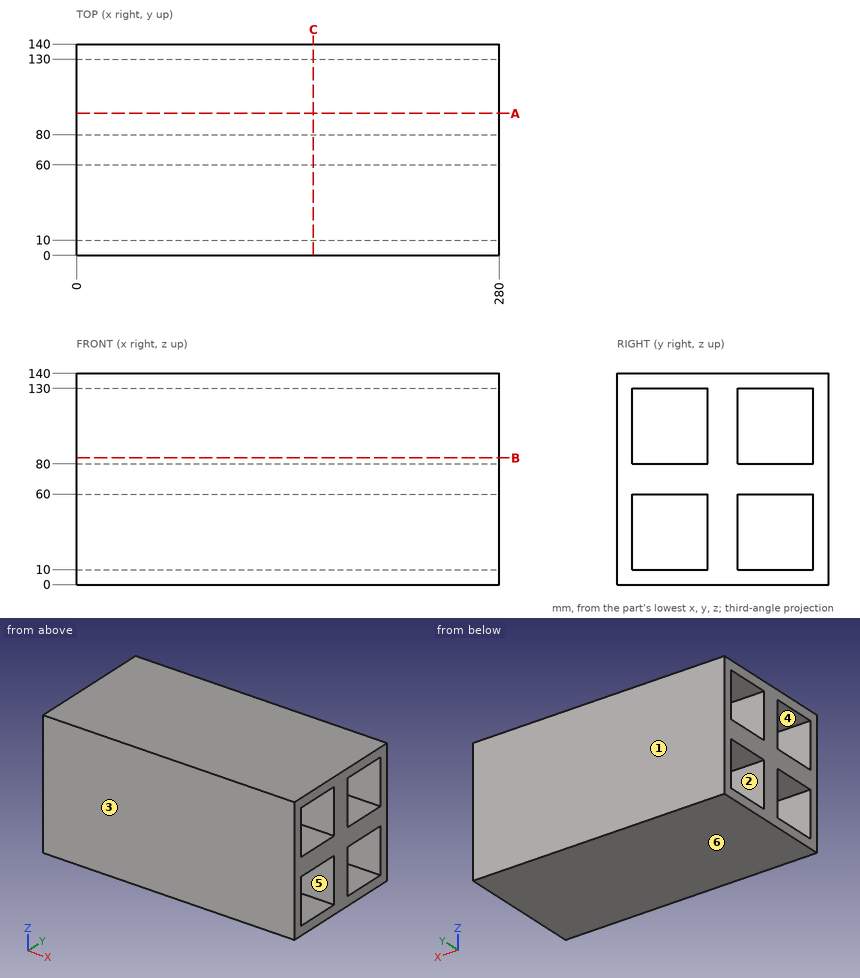
Study the drawing (mm; zero at the part's minimum x, y, z) and answer. A direction names the side the tool comes from. Give positions to 0.01 mm unless a question says otherwise; leave off trailing zeros. Write each loop counter-clockwise with the first axis right and the second up, starting at its lowest first coordinate (ties: lowest second). Pieces come first, ordered by that corner, then holes.
Item 1: Section C-C, the plane x = 157 is taken. Write down the section's boundary in (y, z), plus the area to 3 significant figures.
Item 2: Which of the six approach directions +Z, -Z, +X, -X, +Y, -Y give full straight-line access (tool end or side, diameter ignored) to the marked faces 1 and 2?
Item 3: Section A-A, the plane y = 94 is taken. Write down the section's boundary in (x, z).
Item 4: Determine the mould class of the marked faces 3, 4, 5 and 6 for opening direction Z: released by +Z, released by -Z, zero draft, split by the parting line, or undercut.
Item 5: Find the intervals of material crossed by line 1 along Y through (x, z) = (247.5, 29), in increasing order.
Completed:
1. outline: (0, 0) - (140, 0) - (140, 140) - (0, 140) - close; hole (10, 10) - (60, 10) - (60, 60) - (10, 60) - close; hole (10, 80) - (60, 80) - (60, 130) - (10, 130) - close; hole (80, 10) - (130, 10) - (130, 60) - (80, 60) - close; hole (80, 80) - (130, 80) - (130, 130) - (80, 130) - close
1. area: 9,600 mm2
2. face 1: +Z, -Z, +X, -X, +Y
2. face 2: +X, -X
3. outline: (0, 0) - (280, 0) - (280, 10) - (0, 10) - close; (0, 60) - (280, 60) - (280, 80) - (0, 80) - close; (0, 130) - (280, 130) - (280, 140) - (0, 140) - close
4. face 3: zero draft
4. face 4: undercut
4. face 5: undercut
4. face 6: released by -Z
5. line 1: y = 0 to 10, 60 to 80, 130 to 140
